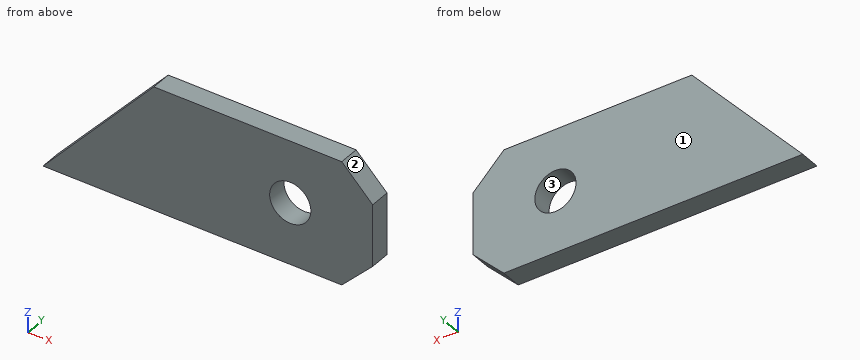
from build123d import *

# Parameters (mm, degrees)
F0_W     = 160
F0_H     = 60
F0_R     = 10
F1_DEPTH = 5
F2_SIZE  = 15
F4_DEPTH = 25


with BuildPart() as f1:
    # F0 (on Front) → F1 (new body, symmetric)
    with BuildSketch(Plane.XZ):
        Rectangle(F0_W, F0_H)
        with Locations((40, 0)):
            Circle(F0_R, mode=Mode.SUBTRACT)
    extrude(amount=F1_DEPTH, both=True)

    # F2
    f2_edges = [f1.edges().sort_by_distance(p)[0] for p in [
        (80, 0, 30),
        (80, 0, -30),
    ]]
    chamfer(f2_edges, length=F2_SIZE)

    # F3 (on face) → F4 (cut)
    with BuildSketch(Plane.XZ.offset(5)):
        Polygon((-80, 30), (-80, -30), (-26.189647, 30), align=None)
    extrude(amount=-F4_DEPTH, mode=Mode.SUBTRACT)


solid = f1.part
The listing builds one solid part. Answer for the finished solid, in the listing's coordinates (mm). Face numbers are marked on the shaded views. Coordinates: 2 decimals unless noted, no trailing zeros. Loops run counter-clockwise (first coordinate to the right, second up) from the corner with the lowest first, then second, coordinate; pieces in that order, holes last. Notation, with made-up numbers: M 26.25,79 L 53.25,79 A18 cw 53.25,104 Z; hole C 67,-21 d3. An arc over 180 degrees is marked long. Answer in a Markdown table with one row per item.
1) Find section B-B (z = 4). Determine the outline of the cut face in (x, y), then the cut area to 3 significant figures.
Answers below:
| item | result |
|---|---|
| outline | M -49.51,-5 L 30.83,-5 L 30.83,5 L -49.51,5 Z; M 49.17,-5 L 80,-5 L 80,5 L 49.17,5 Z |
| area | 1,110 mm^2 |
2) Find the intervals of material crossed by probe 1 along Z at (x, y) = (40, 2.5); probe 2 along X at (y, z) = (-4, -7.5); probe 3 along X at (y, z) = (1, -25), in increasing order.
Answers below:
| item | result |
|---|---|
| probe 1 | -30 to -10, 10 to 30 |
| probe 2 | -59.82 to 33.39, 46.61 to 80 |
| probe 3 | -75.52 to 70 |
3) Find section C-C (y = -0.25). Determine the outline of the cut face in (x, z), then the cut area to 3 significant figures.
Answers below:
| item | result |
|---|---|
| outline | M -80,-30 L 65,-30 L 80,-15 L 80,15 L 65,30 L -26.19,30 Z; hole C 40,0 d20 |
| area | 7,450 mm^2 |
4) Find section A-A (x = 40). Determine the outline of the cut face in (y, z).
Answers below:
| item | result |
|---|---|
| outline | M -5,-30 L 5,-30 L 5,-10 L -5,-10 Z; M -5,10 L 5,10 L 5,30 L -5,30 Z |
5) Find section D-D (x = -68.5). Determine the outline of the cut face in (y, z), then the cut area to 3 significant figures.
Answers below:
| item | result |
|---|---|
| outline | M -5,-30 L 5,-30 L 5,-17.18 L -5,-17.18 Z |
| area | 128 mm^2 |
6) Given pin 1 (5 mm diameter, centred on y = 3, z = -5, fed in from -X); pin 2 (4 mm diameter, centred on y = 2, z = -3.5, fed in from -X); pin 3 (1.5 mm diameter, centred on y = 0, z = 17, fed in from +X), each flat-ended and moving along its own axis, determine where each tip first touches the part or whether it passes through.
Answers below:
| item | result |
|---|---|
| pin 1 | x = -59.82 |
| pin 2 | x = -58.03 |
| pin 3 | x = 78.75 |
7) Determine the mould class of the marked faces 1, 2 and 3 for opening direction X: released by +X, released by -X, zero draft, split by the parting line, or undercut.
Answers below:
| item | result |
|---|---|
| face 1 | zero draft |
| face 2 | released by +X |
| face 3 | undercut |
